For this review, take the finished solid that the model builds, in its own axes (mm). A direction names the side the tool comes from. Give positions to 0.01 mm unless a question says otherwise; leave off trailing zeros. Order: outer loops, then holes, each group sorted by start corner. A loop starts at its lowest first (then second) coordinate and runs counter-clockwise, first axis right, second up.
Item 1: For probe 1 along X at (y, z) = (15, 3.75); probe 2 along Z at (x, y) = (-36, -6), list the stretches that pass through material, from the lowest coordinate up.
Item 2: The part is to be moulded in two halves that separate along Y. For faces 1 (the flat face through (0, 69.85, 4)), 2 (the flat face through (0, 64.62, 5)), 3 (the flat face through (1, 1, 0)), 4 (the flat face through (65, -19.05, 3)), say which applies: released by +Y, released by -Y, zero draft, split by the parting line, or undercut.
Item 3: Consider section A-A (z = 4.75). Give the boundary of the cut face in (x, y), plus the area to 3 significant figures.
Item 4: For P1, Ø6, axis at x = -1.5, y = -42, coming from the +Z side; P2, Ø1.5, axis at y = 25.5, z = 3, coming from the +X side; P3, Ø2.5, axis at x = -64.5, z = 5.5, coming from the -Y side; P4, Ø2.5, axis at x = 62.5, z = 5, coming from the -Y side, all flat-tipped, find the tip position at first contact; note any pin that passes through.
Item 5: Consider section D-D (x = 28.5). Give the boundary of the cut face in (y, z), plus the area to 3 significant figures.
Item 6: Machinability: for faces 5 (the flat face through (-65, -19.05, 3)), 6 (the flat face through (-19.05, 65, 3)), 7 (the flat face through (-64.62, 0, 5)), which of the approach directions +Z, -Z, +X, -X, +Y, -Y give a long, thin tool a straight path to every point of the face, cutting with its end or side? Answer none if there is none.
Item 7: Consider section B-B (y = 1). Give the boundary of the cut face in (x, z).
```python
from build123d import *

# Parameters (mm, degrees)
BOSS_EXTRUDE1_DEPTH = 2.54
SKETCH2_W           = 38.1
SKETCH2_H           = 5.229692412
SKETCH2_W_2         = 5.229692412
SKETCH2_H_2         = 38.1
BOSS_EXTRUDE2_DEPTH = 5.08


with BuildPart() as part:
    # Sketch1 → Boss-Extrude1 (new body)
    with BuildSketch(Plane.XY):
        Polygon((57.15, 19.05), (69.85, 19.05), (69.85, -19.05), (57.15, -19.05), (19.05, -57.15), (19.05, -69.85), (-19.05, -69.85), (-19.05, -57.15), (-57.15, -19.05), (-69.85, -19.05), (-69.85, 19.05), (-57.15, 19.05), (-19.05, 57.15), (-19.05, 69.85), (19.05, 69.85), (19.05, 57.15), align=None)
    extrude(amount=BOSS_EXTRUDE1_DEPTH)

    # Sketch2 → Boss-Extrude2 (add)
    with BuildSketch(Plane.XY.offset(2.54)):
        with Locations((0, -67.235153794)):
            Rectangle(SKETCH2_W, SKETCH2_H)
        with Locations((-67.235153794, 0)):
            Rectangle(SKETCH2_W_2, SKETCH2_H_2)
        with Locations((0, 67.235153794)):
            Rectangle(SKETCH2_W, SKETCH2_H)
        with Locations((67.235153794, 0)):
            Rectangle(SKETCH2_W_2, SKETCH2_H_2)
    extrude(amount=BOSS_EXTRUDE2_DEPTH)


solid = part.part
```
Resolved:
1. probe 1: x = -69.85 to -64.62, 64.62 to 69.85
1. probe 2: z = 0 to 2.54
2. face 1: released by +Y
2. face 2: undercut
2. face 3: zero draft
2. face 4: released by -Y
3. outline: (-69.85, -19.05) - (-64.62, -19.05) - (-64.62, 19.05) - (-69.85, 19.05) - close; (-19.05, -69.85) - (19.05, -69.85) - (19.05, -64.62) - (-19.05, -64.62) - close; (-19.05, 64.62) - (19.05, 64.62) - (19.05, 69.85) - (-19.05, 69.85) - close; (64.62, -19.05) - (69.85, -19.05) - (69.85, 19.05) - (64.62, 19.05) - close
3. area: 797 mm2
4. P1: stops at z = 2.54
4. P2: stops at x = 51.29
4. P3: stops at y = -19.05
4. P4: passes through
5. outline: (-47.7, 0) - (47.7, 0) - (47.7, 2.54) - (-47.7, 2.54) - close
5. area: 242 mm2
6. face 5: +Z, -Z, -X, -Y
6. face 6: +Z, -Z, -X, +Y
6. face 7: +Z, +Y, -Y
7. outline: (-69.85, 0) - (69.85, 0) - (69.85, 7.62) - (64.62, 7.62) - (64.62, 2.54) - (-64.62, 2.54) - (-64.62, 7.62) - (-69.85, 7.62) - close
